```python
from build123d import *

# Parameters (mm, degrees)
F0_W     = 254
F0_H     = 127
F1_DEPTH = 76.2
F4_DEPTH = 76.201
F2_R     = 19.05
F5_DEPTH = 279.4


with BuildPart() as f1:
    # F0 (on Top) → F1 (new body)
    with BuildSketch(Plane.XY):
        with Locations((127, 63.5)):
            Rectangle(F0_W, F0_H)
    extrude(amount=F1_DEPTH)

    # F3 (on Top) → F4 (cut, through all)
    with BuildSketch(Plane.XY):
        with BuildLine():
            add(Edge.make_bspline(
                [(50.8, 38.1), (61.798523, 38.1), (56.299261, 76.2), (50.8, 114.3), (45.300739, 76.2), (39.801477, 38.1), (50.8, 38.1)],
                knots=[0, 0, 0, 2.094395, 2.094395, 4.18879, 4.18879, 6.283185, 6.283185, 6.283185], degree=2, weights=[1, 0.5, 1, 0.5, 1, 0.5, 1]))
        make_face()
    extrude(amount=F4_DEPTH, mode=Mode.SUBTRACT)

    # F2 (on Top) → F5 (cut)
    with BuildSketch(Plane.XY):
        with Locations((184.15, 63.5)):
            Circle(F2_R)
    extrude(amount=F5_DEPTH, mode=Mode.SUBTRACT)


solid = f1.part
```
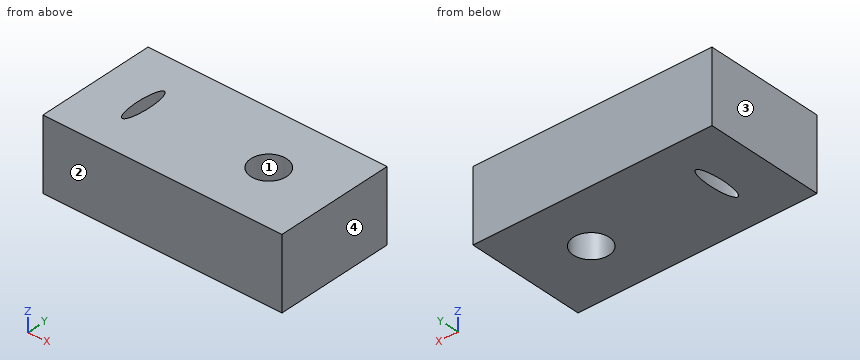
Source: CAD feature listing. Evaluate the final solid. Frame: model axes, mm. Face numbers are marked on the shaded views. Coordinates: 2 decimals unless noted, no trailing zeros. Loops run counter-clockwise (first coordinate to the right, second up) from the corner with the lowest first, then second, coordinate; pieces in that order, holes last. Notation, with made-up numbers: M 11,20 L 59,20 A26 cw 59,53 Z; hole C 65,18 d1. An arc over 180 degrees is marked long. Use a Markdown table: item, result. Add a question column.
Q1. Draft query along X for the marked faces 1, 2, 3 and 4. Return one class per face: pulls with the +X half, pulls with the -X half, needs draft (parallel to the pull), parting line crosses it, or undercut.
Q2. Section query A-A, the plane x = 184.15. Return loops of the section in (y, z), and give its area (3 significant figures).
Q3. Section query B-B, the plane y = 63.5. State how many separate pieces and enclosed holes the cut face has, and give its area (3 significant figures).
Q4. Material intervals for L1, parallel to X at y = 63, z = 42; L2, parallel to Y at x = 184.15, z = 35.5; L3, parallel to X at y = 48, z = 10, sorted ascending.
Result:
| question | item | result |
|---|---|---|
| 1 | face 1 | undercut |
| 1 | face 2 | needs draft |
| 1 | face 3 | pulls with the -X half |
| 1 | face 4 | pulls with the +X half |
| 2 | outline | M 0,0 L 44.45,0 L 44.45,76.2 L 0,76.2 Z; M 82.55,0 L 127,0 L 127,76.2 L 82.55,76.2 Z |
| 2 | area | 6,770 mm2 |
| 3 | separate pieces | 3 |
| 3 | enclosed holes | 0 |
| 3 | area | 15,500 mm2 |
| 4 | L1 | x = 0 to 44.45, 57.15 to 165.11, 203.19 to 254 |
| 4 | L2 | y = 0 to 44.45, 82.55 to 127 |
| 4 | L3 | x = 0 to 45.77, 55.83 to 173.08, 195.22 to 254 |
